Check sheet for the modelled part. Datum: model origin and axes. Units: mm. Face numbers are marked on the shaded views. A direction names the side the tool comes from. Give positions to 0.01 mm unless a question says otherwise; leave off trailing zeros. Order: outer loops, then holes, each group sorted by start corner. A loop starts at its lowest first (then second) coordinate and runs counter-clockwise, first axis right, second up. Notation, with made-up numbers: (18.5, 70.25) -> (48.5, 70.25) arc R17 cw to (48.5, 79.25) -> close; hole circle Ø7 at (-34, 59.5). An arc over 180 degrees is marked (long way). One line per question, with ' | ' between items. Start each with the question number.
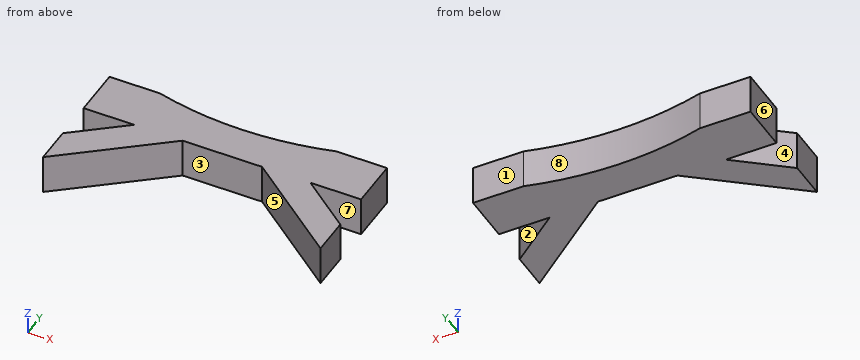
from build123d import *

# Parameters (mm, degrees)
BOSS_EXTRUDE1_DEPTH = 5.08


with BuildPart() as part:
    # Sketch1 → Boss-Extrude1 (new body)
    with BuildSketch(Plane.XY):
        with BuildLine():
            Line((6.468659765, 0), (0, -5.08))
            Line((0, -5.08), (0, -9.924449534))
            Line((0, -9.924449534), (12.637379407, 0))
            Line((12.637379407, 0), (22.797379407, 0))
            Line((22.797379407, 0), (35.434758815, -9.924449534))
            Line((35.434758815, -9.924449534), (35.434758815, -5.08))
            Line((35.434758815, -5.08), (28.96609905, 0))
            Line((28.96609905, 0), (35.434758815, 0))
            Line((35.434758815, 0), (35.434758815, 6.35))
            Line((35.434758815, 6.35), (28.96609905, 6.35))
            ThreePointArc((28.96609905, 6.35), (17.717379407, 4.859071786), (6.468659765, 6.35))
            Line((6.468659765, 6.35), (0, 6.35))
            Line((0, 6.35), (0, 0))
            Line((0, 0), (6.468659765, 0))
        make_face()
    extrude(amount=BOSS_EXTRUDE1_DEPTH)


solid = part.part
1. Go/stop test with flat-tipped pins: pin 1 (2 mm diameter, centred on x = 13.5, z = 2, fed in from +Y); pin 2 (1.5 mm diameter, centred on x = 5, z = 2.5, fed in from -Y); pin 3 (2.5 mm diameter, centred on x = 33.5, z = 2.5, fed in from -Y). Record where each tip stops, or that it passes through.
2. Tool access check on the marked faces 1, 2, 3 and 4. Record the directions out of +Z, -Z, +X, -X, +Y, -Y that give a thin tool (end or side, any length) a straight path to the whole face; none if there is none.
3. Cross-section at C-C on z = 4.4. Record the boundary of the cut face in (x, y), and give its area (3 significant figures).
4. Cross-section at A-A on y = 5.25. Record the boundary of the cut face in (x, z), and give its area (3 significant figures).
5. Cross-section at D-D on x = 15. Record the boundary of the cut face in (y, z).
6. Scan lines: probe 1 along X at (y, z) = (-4, 3.75); probe 2 along Y at (x, z) = (22, 2.3); probe 3 along X at (y, z) = (-7.5, 4). Record each from-to range of solid material in increasing order.
7. Cross-section at B-B on x = 29.5. Record the boundary of the cut face in (y, z), and give its area (3 significant figures).
8. Mould release check, pull along Y, two halves, no side actions. Record for the marked faces 5, 6, 7 and 8: +Y half, -Y half, draft (parallel to the pull), parting line (faces both ways), or undercut.
Response values:
1) pin 1: stops at y = 5.18 | pin 2: stops at y = -6.59 | pin 3: stops at y = -9.39
2) face 1: +Z, -Z, +X, -X, +Y | face 2: +Z, -Z, +X | face 3: +Z, -Z, -Y | face 4: +Z, -Z, -X
3) outline: (0, -9.92) -> (12.64, 0) -> (22.8, 0) -> (35.43, -9.92) -> (35.43, -5.08) -> (28.97, 0) -> (35.43, 0) -> (35.43, 6.35) -> (28.97, 6.35) arc R43.18 cw to (6.47, 6.35) -> (0, 6.35) -> (0, 0) -> (6.47, 0) -> (0, -5.08) -> close | area: 295 mm²
4) outline: (0, 0) -> (11.92, 0) -> (11.92, 5.08) -> (0, 5.08) -> close; (23.51, 0) -> (35.43, 0) -> (35.43, 5.08) -> (23.51, 5.08) -> close | area: 121 mm²
5) outline: (0, 0) -> (4.94, 0) -> (4.94, 5.08) -> (0, 5.08) -> close
6) probe 1: x = 1.38 to 7.54, 27.89 to 34.06 | probe 2: y = 0 to 5.07 | probe 3: x = 0 to 3.09, 32.35 to 35.43
7) outline: (-5.26, 0) -> (-0.42, 0) -> (-0.42, 5.08) -> (-5.26, 5.08) -> close; (0, 0) -> (6.35, 0) -> (6.35, 5.08) -> (0, 5.08) -> close | area: 56.9 mm²
8) face 5: -Y half | face 6: draft | face 7: undercut | face 8: +Y half
